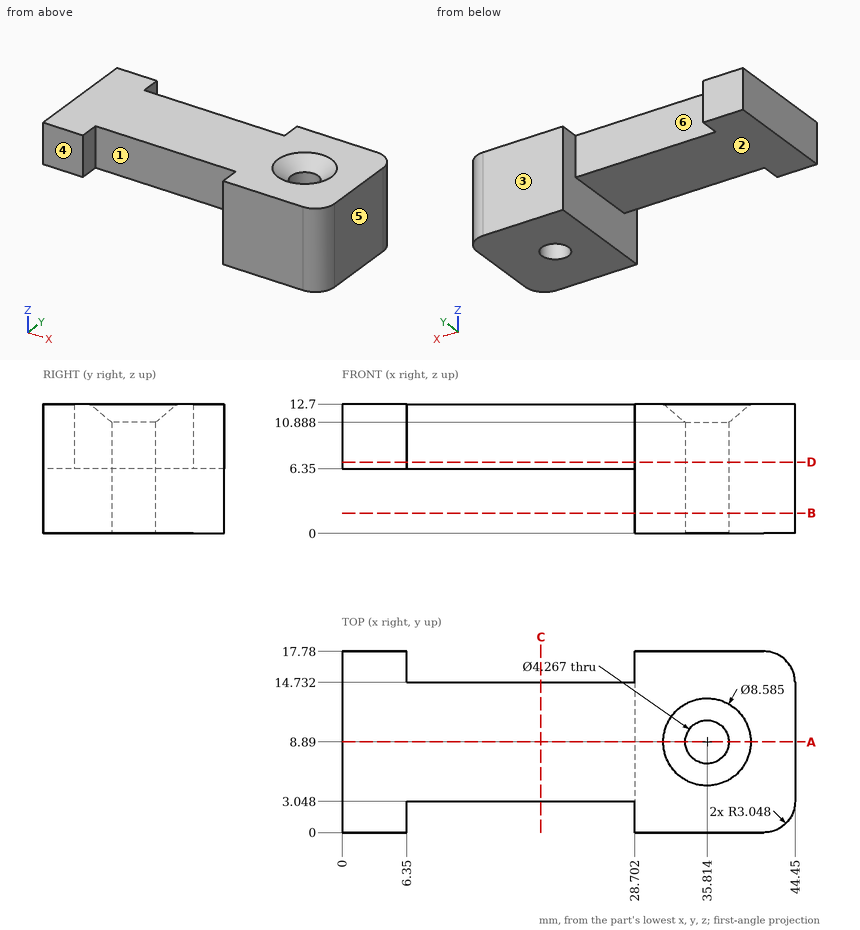
Study the drawing (mm; zero at the part's minimum x, y, z) and answer. A direction names the side the tool comes from. Coordinates: 2 decimals unless noted, no trailing zeros. Loops run counter-clockwise (first coordinate to the right, second up) from the corner with the lowest first, then second, coordinate; pieces in that order, holes last. Notation, with made-up numbers: M 33.5,50.5 L 49.5,50.5 A15 ccw 49.5,62.5 Z; hole C -31.5,-35 d11. An arc over 180 degrees is marked long. Answer in a Markdown table with one row per item.
1) Find section C-C (x = 19.5). Determine the outline of the cut face in (y, z), then the cut area to 3 significant figures.
Answers below:
| item | result |
|---|---|
| outline | M 3.05,6.35 L 14.73,6.35 L 14.73,12.7 L 3.05,12.7 Z |
| area | 74.2 mm^2 |
2) Find section D-D (z = 7). Determine the outline of the cut face in (x, y), then the cut area to 3 significant figures.
Answers below:
| item | result |
|---|---|
| outline | M 0,0 L 6.35,0 L 6.35,3.05 L 28.7,3.05 L 28.7,0 L 41.4,0 A3.05 ccw 44.45,3.05 L 44.45,14.73 A3.05 ccw 41.4,17.78 L 28.7,17.78 L 28.7,14.73 L 6.35,14.73 L 6.35,17.78 L 0,17.78 Z; hole C 35.81,8.89 d4.27 |
| area | 636 mm^2 |
3) Determine the mould class of the marked faces 4, 5 and 6 for opening direction X: released by +X, released by -X, zero draft, split by the parting line, or undercut.
Answers below:
| item | result |
|---|---|
| face 4 | zero draft |
| face 5 | released by +X |
| face 6 | undercut |
4) Find the intervals of material crossed by probe 1 along X at (y, z) = (8.89, 4); probe 2 along Y at (x, z) = (22, 10.5); probe 3 along X at (y, z) = (12.25, 3.75), in increasing order.
Answers below:
| item | result |
|---|---|
| probe 1 | 28.7 to 33.68, 37.95 to 44.45 |
| probe 2 | 3.05 to 14.73 |
| probe 3 | 28.7 to 44.45 |
5) Which of the six approach directions +Z, -Z, +X, -X, +Y, -Y give full straight-line access (tool end or side, diameter ignored) to the marked faces 1, 2 and 3?
Answers below:
| item | result |
|---|---|
| face 1 | +Z, -Z, -Y |
| face 2 | -Z, -X, +Y, -Y |
| face 3 | +Z, -Z, +X, -X, +Y |
6) Find section B-B (z = 2). Determine the outline of the cut face in (x, y).
Answers below:
| item | result |
|---|---|
| outline | M 28.7,0 L 41.4,0 A3.05 ccw 44.45,3.05 L 44.45,14.73 A3.05 ccw 41.4,17.78 L 28.7,17.78 Z; hole C 35.81,8.89 d4.27 |
7) Given pin 1 (2.5 mm diameter, centred on y = 1.5, z = 8, fed in from +X) (1 decimal); pin 2 (5 mm diameter, centred on x = 22, z = 10.5, fed in from +Y); pin 3 (5 mm diameter, centred on x = 35.814, y = 8.89, fed in from +Z) (1 decimal), each flat-ended and moving along its own axis, determine where each tip first touches the part or whether it passes through.
Answers below:
| item | result |
|---|---|
| pin 1 | x = 44.4 |
| pin 2 | y = 14.73 |
| pin 3 | z = 11.2 |
8) Find section A-A (y = 8.89). Determine the outline of the cut face in (x, z), then the cut area to 3 significant figures.
Answers below:
| item | result |
|---|---|
| outline | M 0,6.35 L 28.7,6.35 L 28.7,0 L 33.68,0 L 33.68,10.89 L 31.52,12.7 L 0,12.7 Z; M 37.95,0 L 44.45,0 L 44.45,12.7 L 40.11,12.7 L 37.95,10.89 Z |
| area | 324 mm^2 |
